Check sheet for the drawn part. Datum: minimum x, y, z corner. Units: mm. Give positions to 0.01 mm unless a question says otherwise; leave off trailing zeros. Write each loop counter-clockwise with the first axis right and the second up, starting at its lowest first coordinate (ties: lowest second). Pieces come first, ordered by that corner, then holes. Notation, with made-up numbers: (-16.5, -13.75) - (-2.5, -13.75) arc R15 ccw to (-2.5, 8.25) - close; hole circle Ø11 at (-17, 6). An arc over 180 degrees is marked (long way). Answer as a JSON object with one key per item and string values. Group by question number.
Item 1: Go/stop test with flat-tipped pins: pin 1 (4 mm diameter, centred on x = 12.5, y = 6, fed in from -Z); pin 2 (2 mm diameter, centred on x = 12.5, y = 3, fed in from +Z). Record where each tip stops, or that it passes through.
Item 2: Scan lines: line 1 along Y through (x, z) = (4.25, 18); line 2 along Z through (x, y) = (8, 4); line 3 along X through (y, z) = (9.5, 1.75). Record each from-to range of solid material in increasing order. Write a range as [from, to].
Item 3: Sectioned sample at B-B, the plane x = 9. Record the boundary of the cut face in (y, z).
Item 4: Sectioned sample at A-A, the plane z = 5.5. Record the boundary of the cut face in (x, y), and give its area (3 significant figures).
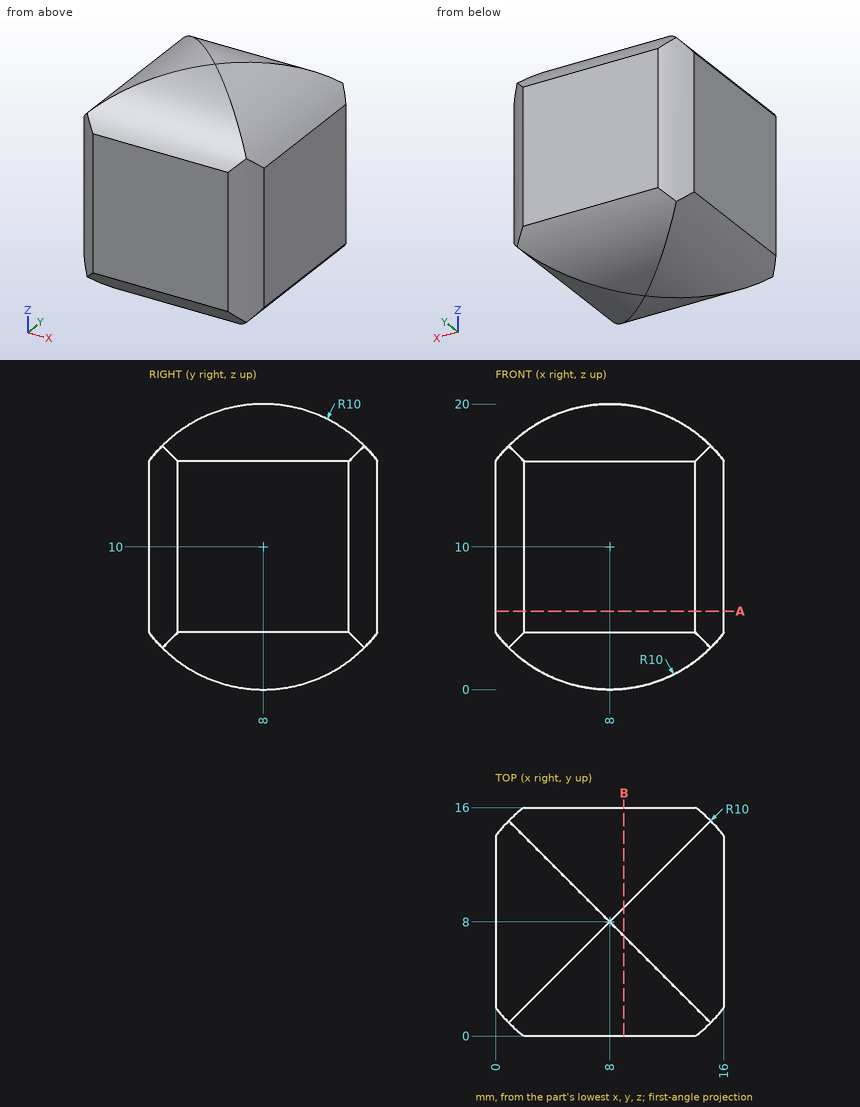
Geometry check:
{
 "1": {"pin 1": "z = 0.32", "pin 2": "z = 19.13"},
 "2": {"line 1": "[2, 14]", "line 2": "[0.83, 19.17]", "line 3": "[2.35, 13.65]"},
 "3": {"outline": "(0, 4) arc R10 ccw to (7, 0.05) - (9, 0.05) arc R10 ccw to (16, 4) - (16, 16) arc R10 ccw to (9, 19.95) - (7, 19.95) arc R10 ccw to (0, 16) - close"},
 "4": {"outline": "(0, 2) arc R10 ccw to (2, 0) - (14, 0) arc R10 ccw to (16, 2) - (16, 14) arc R10 ccw to (14, 16) - (2, 16) arc R10 ccw to (0, 14) - close", "area": "249 mm^2"}
}
